Geometry: final body of the model. Coordinates: model frame, mm. Face numbers are marked on the shaded views. A direction names the side the tool comes from. Give positions to 0.01 mm unless a question says otherwise; leave off trailing zeros. Write each loop counter-clockwise with the first axis right and the second up, starting at its lowest first coordinate (ties: lowest second). Pieces come first, ordered by that corner, then holes. Notation, with made-up numbers: (-5, -40) -> (4, -40) arc R20 cw to (4, -32) -> close; hole circle Ø9 at (81.25, 38). An arc over 180 degrees is marked (long way). Answer in a Markdown table with one row per item. Add a question column.
Item 1: Section query A-A on x = 72.7. Output: boundary loops of the cut face in (y, z).
Item 2: Section query D-D on x = 328.5. Output: boundary loops of the cut face in (y, z).
Item 3: Access query for the marked faces 1 and 2. Directions: +Z, -Z, +X, -X, +Y, -Y. A direction counts if a zero-diameter tool reaches every point of the face in a straight line with its end or side. Return the directions, or none.
Item 4: Section query B-B on z = 88.9. Output: boundary loops of the cut face in (x, y) (1 decimal).
Item 5: Section query C-C on z = 111.5. Output: boundary loops of the cut face in (x, y) (3 decimals).
Item 6: Material intervals for probe 1 along X at (y, z) = (11.5, 149) (3 decimals); probe 2 along Z at (x, y) = (177.5, 2); probe 3 along X at (y, z) = (2, 20.5) (3 decimals), sorted ascending. Write a range as from..to.
Item 7: First-contact query: P1, Ø2.5, axis at x = 390.525, z = 171.45, coming from the +Y side; P2, Ø2, axis at y = 3.5, z = 96, coming from the +X side; P3, Ø3.5, axis at y = 1.5, z = 122, coming from the -X side; P4, Ø5, axis at x = 105, z = 142, coming from the +Y side. Flat tips, straight axial feed; report the tip coordinate or a pass-through.
Autodesk Inventor part; units mm, degrees
ref_plane "YZ Plane" through (0, 0, 0) normal (1, 0, 0) x (0, 1, 0)
ref_plane "XZ Plane" through (0, 0, 0) normal (0, 1, 0) x (-1, 0, 0)
ref_plane "XY Plane" through (0, 0, 0) normal (0, 0, 1) x (1, 0, 0)
sketch "Sketch1" plane through (0, 0, 0) normal (0, 1, 0) x (-1, 0, 0)
  line L0 (0, 0) -> (-428.625, 0)
  line L1 (-428.625, 0) -> (-428.625, 177.8)
  line L2 (-428.625, 177.8) -> (0, 177.8)
  line L3 (0, 177.8) -> (0, 0)
  dimension "d0" = 428.625
  dimension "d1" = 177.8
extrude "Plate1" add sketch "Sketch1" along normal blind 3.048
sketch "Sketch2" plane through (3.048, 0, 177.8) normal (-1, 0, 0) x (0, -1, 0)
  line L0 (0, -177.8) -> (0, 0)
  line L1 (0, 0) -> (-12.7, 0)
  line L2 (-12.7, 0) -> (-12.7, -177.8)
  line L3 (-12.7, -177.8) -> (0, -177.8)
edge flange "Flange1" height 12.7 angle 90 thickness 3.048 bend radius 3.048 thickness toward (-1, 0, 0) relief straight relief width 3.048 relief depth 1.524 corner gap 3.048 corner form 0 edges at (0, 3.048, 88.9) (428.625, 3.048, 88.9) wall of the first edge with corners at (3.048, 0, 0) (3.048, 0, 177.8) (3.048, 12.7, 177.8) (3.048, 12.7, 0)
bend "Bend1"
corner "Corner1"
sketch "Sketch3" plane through (0, 12.7, 0) normal (-1, 0, 0) x (0, 0, 1)
  line L0 (0, -6.604) -> (0, 0)
  line L1 (0, 0) -> (177.8, 0)
  line L2 (177.8, -12.7) -> (0, -12.7)
  line L3 (177.8, 0) -> (177.8, -6.604)
  line L4 (4.7625, -4.445) -> (173.0375, -4.445) construction
  line L5 (88.9, 0) -> (88.9, -12.7) construction
  dimension "d13" = 168.275
  dimension "d14" = 4.445
hole "Hole1" at (0, 8.255, 4.7625) at (0, 8.255, 173.0375) direction (1, 0, 0) diameter 4 end through all
sketch "Sketch4" plane through (0, 0, 0) normal (0, -1, 0) x (1, 0, 0)
  line L0 (428.625, 177.8) -> (428.625, 0)
  line L1 (0, 0) -> (0, 177.8)
  line L2 (422.529, 177.8) -> (6.096, 177.8)
  line L3 (6.096, 0) -> (422.529, 0)
  line L4 (422.529, 0) -> (422.529, 177.8)
  line L5 (396.875, 158.75) -> (415.925, 158.75)
  line L6 (415.925, 158.75) -> (415.925, 19.05)
  line L7 (415.925, 19.05) -> (396.875, 19.05)
  line L8 (396.875, 19.05) -> (396.875, 158.75)
  dimension "d22" = 31.75
  dimension "d23" = 19.05
  dimension "d24" = 19.05
  dimension "d25" = 19.05
extrude "Cut1" cut sketch "Sketch4" against normal blind 3.048
sketch "Sketch5" plane through (0, 0, 0) normal (0, -1, 0) x (1, 0, 0)
  line L0 (422.529, 177.8) -> (6.096, 177.8)
  line L1 (6.096, 177.8) -> (6.096, 0) construction
  line L2 (6.096, 0) -> (422.529, 0)
  line L3 (422.529, 0) -> (422.529, 177.8)
  line L4 (12.446, 171.45) -> (390.525, 171.45) construction
  line L5 (390.525, 171.45) -> (390.525, 6.35) construction
  line L6 (390.525, 6.35) -> (12.446, 6.35) construction
  line L7 (12.446, 6.35) -> (12.446, 171.45) construction
  line L8 (396.875, 19.05) -> (396.875, 158.75)
  point P0 (0, 0)
  dimension "d28" = 6.35
  dimension "d29" = 6.35
  dimension "d30" = 6.35
  dimension "d31" = 6.35
hole "Hole2" at (12.446, 0, 171.45) at (12.446, 0, 6.35) at (390.525, 0, 6.35) at (390.525, 0, 171.45) direction (0, 1, 0) diameter 3 end through all
sketch "Sketch6" plane through (0, 0, 0) normal (0, -1, 0) x (1, 0, 0)
  line L0 (422.529, 177.8) -> (6.096, 177.8)
  line L1 (6.096, 177.8) -> (6.096, 0)
  line L2 (422.529, 0) -> (422.529, 177.8)
  line L3 (6.096, 0) -> (422.529, 0)
  circle A0 centre (72.7, 88.9) radius 60
  circle A1 centre (201.2875, 88.9) radius 60
  circle A2 centre (329.875, 88.9) radius 60
  line L4 (72.7, 88.9) -> (329.875, 88.9) construction
  line L5 (12.7, 177.8) -> (12.7, 0) construction
  line L6 (0, 0) -> (0, 177.8)
  dimension "d39" = 120
  dimension "d40" = 120
  dimension "d41" = 120
  dimension "d42" = 257.175
  dimension "d43" = 128.5875
  dimension "d44" = 177.8
  dimension "d45" = 88.9
  dimension "d46" = 12.7
extrude "Cut2" cut sketch "Sketch6" against normal blind 3.048 contours A0 | A1
sketch "Sketch8" plane through (0, 0, 0) normal (0, -1, 0) x (1, 0, 0)
  line L0 (422.529, 177.8) -> (6.096, 177.8)
  line L1 (422.529, 177.8) -> (6.096, 177.8)
  line L2 (270.129, 177.8) -> (422.529, 177.8)
  line L3 (422.529, 177.8) -> (422.529, 184.15)
  line L4 (422.529, 184.15) -> (270.129, 184.15)
  line L5 (270.129, 184.15) -> (270.129, 177.8)
  point P0 (0, 0)
  dimension "d55" = 6.35
  dimension "d56" = 152.4
sheet face with bend "Face2" sketch "Sketch8" thickness 3.048 toward (0, 1, 0) bend radius 3.048
bend "Bend2"
sketch "Sketch7" plane through (0, 0, 0) normal (0, -1, 0) x (1, 0, 0)
  line L0 (422.529, 177.8) -> (6.096, 177.8) construction
  line L1 (6.096, 0) -> (422.529, 0) construction
  line L2 (396.875, 19.05) -> (396.875, 158.75) construction
  line L3 (276.225, 179.375) -> (377.825, 179.375) construction
  line L4 (377.825, 179.375) -> (377.825, 4.775) construction
  line L5 (377.825, 4.775) -> (276.225, 4.775) construction
  line L6 (276.225, 4.775) -> (276.225, 179.375) construction
  line L7 (276.225, 92.075) -> (377.825, 92.075) construction
  point P0 (0, 0)
  dimension "d49" = 101.6
  dimension "d50" = 174.6
  dimension "d51" = 177.8
  dimension "d52" = 85.725
  dimension "d53" = 19.05
hole "Hole3" at (276.225, 0, 179.375) at (377.825, 0, 179.375) at (377.825, 0, 4.775) at (276.225, 0, 4.775) at (276.225, 0, 179.375) direction (0, 1, 0) diameter 3 end through all
fillet "Corner Round1" radius 3.175 3 edges at (270.129, 1.524, 184.15) (270.129, 1.524, 177.8) (422.529, 1.524, 184.15)
equation "\"d20\" = Thickness"
equation "\"d25\" = d24"
equation "\"d26\" = Thickness"
equation "\"d29\" = d28"
equation "\"d30\" = d28"
equation "\"d31\" = d28"
equation "\"d37\" = Thickness"
equation "\"d43\" = 0.5 * d42"
equation "\"d45\" = 0.5 * d44"
equation "\"d47\" = Thickness"
equation "\"d67\" = Thickness"
equation "\"d2\" = Thickness"
equation "\"d3\" = BendReliefWidth"
equation "\"d4\" = BendReliefDepth"
equation "\"d5\" = MinimumRemnant"
equation "\"d6\" = TransitionRadius"
equation "\"d9\" = BendRadius"
equation "\"d10\" = CornerReliefSize"
equation "\"d11\" = GapSize"
equation "\"d12\" = JacobiRadiusSize"
equation "\"d57\" = BendRadius"
equation "\"d58\" = BendReliefWidth"
equation "\"d60\" = MinimumRemnant"
equation "\"d59\" = BendReliefDepth"
equation "\"d61\" = TransitionRadius"
equation "\"BendRadius\" = Thickness"
equation "\"BendReliefWidth\" = Thickness"
equation "\"BendReliefDepth\" = 0.5 * Thickness"
equation "\"CornerReliefSize\" = 4 * Thickness"
equation "\"MinimumRemnant\" = 2 * Thickness"
equation "\"TransitionRadius\" = BendRadius"
equation "\"JacobiRadiusSize\" = Thickness"
equation "\"GapSize\" = Thickness"
properties part number "Plate"
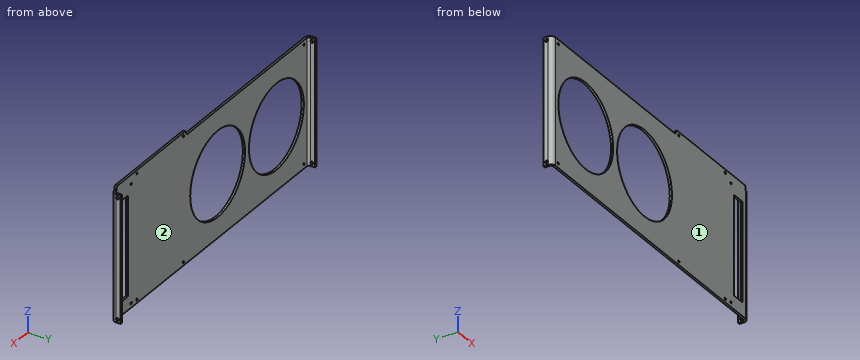
Findings below:
| question | item | result |
|---|---|---|
| 1 | outline | (0, 0) -> (3.05, 0) -> (3.05, 28.9) -> (0, 28.9) -> close; (0, 148.9) -> (3.05, 148.9) -> (3.05, 177.8) -> (0, 177.8) -> close |
| 2 | outline | (0, 0) -> (3.05, 0) -> (3.05, 184.15) -> (0, 184.15) -> close |
| 3 | face 1 | +Z, -Z, +X, -X, -Y |
| 3 | face 2 | +Z, -Z, +Y |
| 4 | outline | (0, 6.1) arc R6.1 ccw to (6.1, 0) -> (12.7, 0) -> (12.7, 3) -> (6.1, 3) arc R3 cw to (3, 6.1) -> (3, 12.7) -> (0, 12.7) -> close; (132.7, 0) -> (141.3, 0) -> (141.3, 3) -> (132.7, 3) -> close; (261.3, 0) -> (396.9, 0) -> (396.9, 3) -> (261.3, 3) -> close; (415.9, 0) -> (422.5, 0) arc R6.1 ccw to (428.6, 6.1) -> (428.6, 12.7) -> (425.6, 12.7) -> (425.6, 6.1) arc R3 cw to (422.5, 3) -> (415.9, 3) -> close |
| 5 | outline | (0, 6.096) arc R6.096 ccw to (6.096, 0) -> (17.119, 0) -> (17.119, 3.048) -> (6.096, 3.048) arc R3.048 cw to (3.048, 6.096) -> (3.048, 12.7) -> (0, 12.7) -> close; (128.281, 0) -> (145.707, 0) -> (145.707, 3.048) -> (128.281, 3.048) -> close; (256.868, 0) -> (396.875, 0) -> (396.875, 3.048) -> (256.868, 3.048) -> close; (415.925, 0) -> (422.529, 0) arc R6.096 ccw to (428.625, 6.096) -> (428.625, 12.7) -> (425.577, 12.7) -> (425.577, 6.096) arc R3.048 cw to (422.529, 3.048) -> (415.925, 3.048) -> close |
| 6 | probe 1 | x = 0..3.048, 425.577..428.625 |
| 6 | probe 2 | z = 0..33.82, 143.98..177.8 |
| 6 | probe 3 | x = 1.581..396.875, 415.925..427.044 |
| 7 | P1 | passes through |
| 7 | P2 | stops at x = 428.41 |
| 7 | P3 | stops at x = 0.71 |
| 7 | P4 | stops at y = 3.05 |
